The figure shows three views and two pictorial views of one solid part (mm, origin at its lowest corner). Answer the questions. A direction names the side the tool comes from. Give positions to 0.01 mm unless a question says otherwise; leave off trailing zeros. Order: outer loops, then holes, each group sorted by start corner. A loop starts at its lowest first (then second) coordinate and runs counter-clockwise, first axis right, second up. Notation, with made-up numbers: (0, -29) -> (37, -29) arc R19 cw to (37, -23) -> close; hole circle Ø2 at (66, 29.25). An arc over 180 degrees is marked (long way). One line per item, written item: value. Start each with the question number.
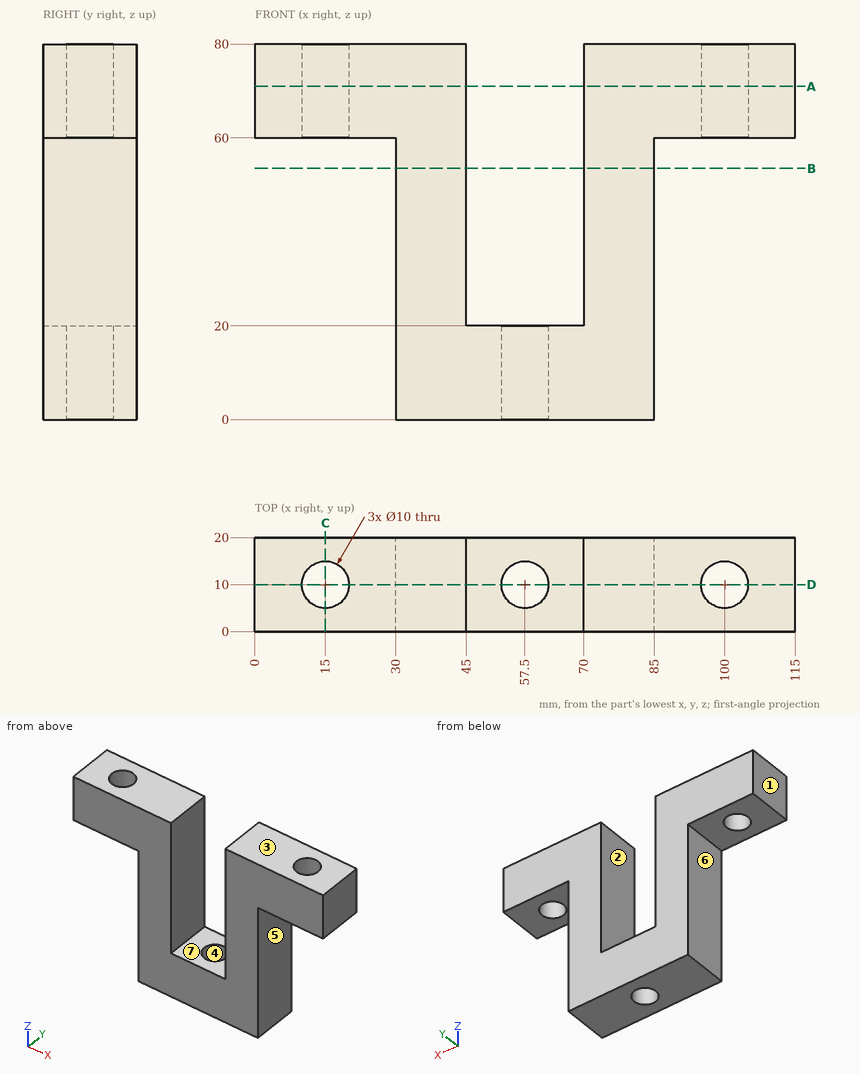
Item 1: Find section B-B on z = 53.5. Write down the section's boundary in (x, y).
Item 2: Find section C-C on x = 15. Write down the section's boundary in (y, z).
Item 3: Find section A-A on z = 71. Write down the section's boundary in (x, y).
Item 4: Flat-ended cylindrical pins translate along their axes: pin 1 (10 mm diameter, centred on x = 93, y = 12, fed in from -Z); pin 2 (10 mm diameter, centred on x = 59.5, y = 10.5, fed in from +Z); pin 3 (5 mm diameter, centred on y = 13, z = 27.5, fed in from +X). Find the tip coordinate at first contact, or state that the pin passes through.
Item 5: Find section D-D on y = 10. Write down the section's boundary in (x, z).
Item 6: Find the intervals of material crossed by line 1 (Y direction, x = 57.5, z = 7.5); line 2 (X direction, y = 13, z = 50); line 3 (X direction, y = 1, z = 69), in increasing order. Write a range as from..to.
Item 7: A tool of negligible diameter and unlimited length cuts with its end or side. For the marked faces 5, 6 and 7, from which of +Z, -Z, +X, -X, +Y, -Y can it reach the whole face along a straight path? Write none if from no direction.
Item 8: For a pull along X with two mould halves and no side action, classify the marked faces 1, 2, 3 and 4 as +X half, -X half, draft (parallel to the pull), parting line (faces both ways), or undercut.
Checks:
1. outline: (30, 0) -> (45, 0) -> (45, 20) -> (30, 20) -> close; (70, 0) -> (85, 0) -> (85, 20) -> (70, 20) -> close
2. outline: (0, 60) -> (5, 60) -> (5, 80) -> (0, 80) -> close; (15, 60) -> (20, 60) -> (20, 80) -> (15, 80) -> close
3. outline: (0, 0) -> (45, 0) -> (45, 20) -> (0, 20) -> close; (70, 0) -> (115, 0) -> (115, 20) -> (70, 20) -> close; hole circle Ø10 at (15, 10); hole circle Ø10 at (100, 10)
4. pin 1: z = 60
4. pin 2: z = 20
4. pin 3: x = 85
5. outline: (0, 60) -> (10, 60) -> (10, 80) -> (0, 80) -> close; (20, 60) -> (30, 60) -> (30, 0) -> (52.5, 0) -> (52.5, 20) -> (45, 20) -> (45, 80) -> (20, 80) -> close; (62.5, 0) -> (85, 0) -> (85, 60) -> (95, 60) -> (95, 80) -> (70, 80) -> (70, 20) -> (62.5, 20) -> close; (105, 60) -> (115, 60) -> (115, 80) -> (105, 80) -> close
6. line 1: 0..5, 15..20
6. line 2: 30..45, 70..85
6. line 3: 0..45, 70..115
7. face 5: -Z, +X, +Y, -Y
7. face 6: -Z, -X, +Y, -Y
7. face 7: +Z, +Y, -Y
8. face 1: -X half
8. face 2: undercut
8. face 3: draft
8. face 4: undercut
